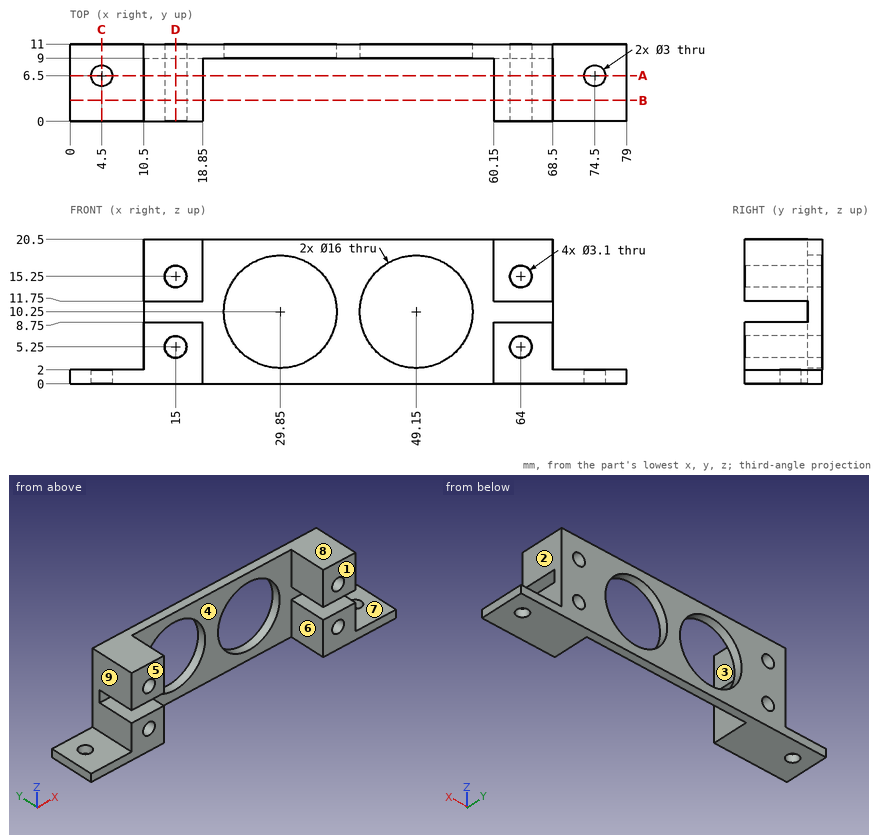
Geometry: see drawing. Coordinates: mm, zero at the bounding-box minimum. A direction names the side the tool comes from. Coordinates: 2 decimals unless noted, no trailing zeros. Loops run counter-clockwise (first coordinate to the right, second up) from the corner with the lowest first, then second, coordinate; pieces in that order, holes last.
Q1. Contact query for flat-ended pins moving along their axis: pin 1 (1.5 mm diameter, centred on y = 9.5, z = 5, fed in from -X); pin 2 (6 mm diameter, centred on y = 5.5, z = 11, fed in from +X); pin 3 (10 mm diameter, centred on x = 46.5, z = 15, fed in from -Y). Output: stop coordinate, or through.
Q2. Set-up query: the marked faces 5, 6, 7, 8 and 9. Return all of +Z, -Z, +X, -X, +Y, -Y with unobstructed straight access to the full face (end or side cutting, diameter ignored); none if empty.
Q3. Draft query along X for the marked faces 1, 2, 3 and 4. Return one class per face: +X half, -X half, draft (parallel to the pull), parting line (faces both ways), or undercut.
Q4. Cut plane B-B (y = 3). Output: boundary loops of the cut face in (x, z), then the cut area to 3 significant figures.
Q5. Cut plane D-D (x = 15). Output: boundary loops of the cut face in (y, z), then the cut area to 3 significant figures.
Q6. Cut plane A-A (y = 6.5). Give the number of separate pieces and of enclosed holes in the cut face, then the cut area to 3 significant figures.
Q7. Cut plane C-C (x = 4.5). Output: boundary loops of the cut face in (y, z), then the cut area to 3 significant figures.
Q8. Material intervals for line 1 (X direction, y = 5.75, z = 5.25); line 2 (X direction, y = 10.2, z = 10.25); line 3 (X direction, y = 9.5, z = 13), sorted ascending.
Working result:
1. pin 1: stops at x = 10.5
1. pin 2: stops at x = 68.5
1. pin 3: stops at y = 9
2. face 5: +Z, -Z, +X, -X, -Y
2. face 6: +Z, -Z, -Y
2. face 7: +Z, +X, +Y, -Y
2. face 8: +Z, +X, -X, +Y, -Y
2. face 9: +Z, -X, +Y, -Y
3. face 1: draft
3. face 2: +X half
3. face 3: undercut
3. face 4: undercut
4. outline: (0, 0) - (18.85, 0) - (18.85, 8.75) - (10.5, 8.75) - (10.5, 2) - (0, 2) - close; (10.5, 11.75) - (18.85, 11.75) - (18.85, 20.5) - (10.5, 20.5) - close; (60.15, 0) - (79, 0) - (79, 2) - (68.5, 2) - (68.5, 8.75) - (60.15, 8.75) - close; (60.15, 11.75) - (68.5, 11.75) - (68.5, 20.5) - (60.15, 20.5) - close; hole circle Ø3.1 at (15, 5.25); hole circle Ø3.1 at (15, 15.25); hole circle Ø3.1 at (64, 5.25); hole circle Ø3.1 at (64, 15.25)
4. area: 304 mm2
5. outline: (0, 0) - (11, 0) - (11, 3.7) - (0, 3.7) - close; (0, 6.8) - (11, 6.8) - (11, 13.7) - (0, 13.7) - (0, 11.75) - (9, 11.75) - (9, 8.75) - (0, 8.75) - close; (0, 16.8) - (11, 16.8) - (11, 20.5) - (0, 20.5) - close
5. area: 130 mm2
6. separate pieces: 6
6. enclosed holes: 4
6. area: 292 mm2
7. outline: (0, 0) - (5, 0) - (5, 2) - (0, 2) - close; (8, 0) - (11, 0) - (11, 2) - (8, 2) - close
7. area: 16.0 mm2
8. line 1: x = 10.5 to 13.45, 16.55 to 18.85, 60.15 to 62.45, 65.55 to 68.5
8. line 2: x = 10.5 to 21.85, 37.85 to 41.15, 57.15 to 68.5
8. line 3: x = 10.5 to 22.34, 37.36 to 41.64, 56.66 to 68.5
